Here's how the part is built. I have some questions about the finished solid (model axes, mm). A direction names the side the tool comes from. Give positions to 0.01 mm unless a question says otherwise; leave off trailing zeros. Loops run counter-clockwise (first coordinate to the right, second up) from the corner with the lowest first, then second, coordinate; pieces in that order, holes last. Notation, with made-up numbers: (6, -13.5) - (30, -13.5) arc R17 cw to (30, 18.5) - close; hole circle Ø4 at (15, 1.5). An arc over 180 degrees is marked (long way). Use a Markdown table: item, result.
from build123d import *

# Parameters (mm, degrees)
PAD_DEPTH       = 10
SKETCH001_R     = 2.5
POCKET_DEPTH    = 6.301
POCKET001_DEPTH = 4.5


with BuildPart() as part:
    # Sketch → Pad (new body, symmetric)
    with BuildSketch(Plane.XZ):
        Polygon((-6.5, 0), (-6.5, 3.2), (-5, 3.2), (-5, 6.3), (5, 6.3), (5, 3.2), (6.5, 3.2), (6.5, 0), (0, 0), align=None)
    extrude(amount=PAD_DEPTH, both=True)

    # Sketch001 (on Face4 of Pad) → Pocket (cut, through all)
    with BuildSketch(Plane(origin=(0, 0, 6.3), x_dir=(-1, 0, 0), z_dir=(0, 0, 1))):
        Circle(SKETCH001_R)
    extrude(amount=-POCKET_DEPTH, mode=Mode.SUBTRACT)

    # Sketch002 (on Face9 of Pocket) → Pocket001 (cut)
    with BuildSketch(Plane(origin=(0, 0, 6.3), x_dir=(-1, 0, 0), z_dir=(0, 0, 1))):
        Polygon((-4.05, 2.338269), (-4.05, -2.338269), (0, -4.676537), (4.05, -2.338269), (4.05, 2.338269), (0, 4.676537), align=None)
    extrude(amount=-POCKET001_DEPTH, mode=Mode.SUBTRACT)


solid = part.part
(1) If I drill on line 1 (X direction, y = -1.25, z = 4); line 2 (X direction, y = 0, z = 1.2); line 3 (Y direction, x = 0, z = 1.2), over which ranges is the centre line in solid material (lowest first)?
A:
| item | result |
|---|---|
| line 1 | -5 to -4.05, 4.05 to 5 |
| line 2 | -6.5 to -2.5, 2.5 to 6.5 |
| line 3 | -10 to -2.5, 2.5 to 10 |
(2) Suppose I cut it at B-B on y = -2. Write out the boundary of the cut face in (x, z), plus the area to 4 significant figures.
A:
| item | result |
|---|---|
| outline | (-6.5, 0) - (-1.5, 0) - (-1.5, 1.8) - (-4.05, 1.8) - (-4.05, 6.3) - (-5, 6.3) - (-5, 3.2) - (-6.5, 3.2) - close; (1.5, 0) - (6.5, 0) - (6.5, 3.2) - (5, 3.2) - (5, 6.3) - (4.05, 6.3) - (4.05, 1.8) - (1.5, 1.8) - close |
| area | 30.75 mm2 |
(3) Will these pins go through, and if not, where does the flat tip stop? pin 1 (1.5 mm diameter, centred on y = -0.5, z = 4, fed in from +X); pin 2 (3.5 mm diameter, centred on y = 2.5, z = 5.5, fed in from -X); pin 3 (2.5 mm diameter, centred on x = 0, y = -2, fed in from +Z).
A:
| item | result |
|---|---|
| pin 1 | x = 5 |
| pin 2 | x = -5 |
| pin 3 | z = 1.8 |
(4) On a 3-axis mill with a long thin cutter (end or side, diameter ignored), from which of +Z, -Z, +X, -X, +Y, -Y can I reach the whole of each face in a straight line? I mean faces 1 (the face through (-2, 3.52, 4.08)), 2 (the face through (5, 0, 5)), 3 (the face through (-5, 0, 5)). Say none if no direction works.
A:
| item | result |
|---|---|
| face 1 | +Z |
| face 2 | +Z, +X, +Y, -Y |
| face 3 | +Z, -X, +Y, -Y |
(5) Suppose I cut it at D-D on x = -2. Write out the boundary of the cut face in (y, z).
A:
| item | result |
|---|---|
| outline | (-10, 0) - (-1.5, 0) - (-1.5, 1.8) - (-3.52, 1.8) - (-3.52, 6.3) - (-10, 6.3) - close; (1.5, 0) - (10, 0) - (10, 6.3) - (3.52, 6.3) - (3.52, 1.8) - (1.5, 1.8) - close |
(6) Suppose I cut it at C-C on y = -6. Write out the boundary of the cut face in (x, z).
A:
| item | result |
|---|---|
| outline | (-6.5, 0) - (6.5, 0) - (6.5, 3.2) - (5, 3.2) - (5, 6.3) - (-5, 6.3) - (-5, 3.2) - (-6.5, 3.2) - close |
(7) Suppose I cut it at A-A on z = 4. Write out the boundary of the cut face in (x, y).
A:
| item | result |
|---|---|
| outline | (-5, -10) - (5, -10) - (5, 10) - (-5, 10) - close; hole (-4.05, -2.34) - (0, -4.68) - (4.05, -2.34) - (4.05, 2.34) - (0, 4.68) - (-4.05, 2.34) - close |
